Check sheet for the drawn part. Datum: minimum x, y, z corner. Units: mm. Give positions to 0.01 mm unless a question says otherwise; leave off trailing zeros. Loops run counter-clockwise (first coordinate to the right, second up) from the corner with the lowest first, then second, coordinate; pieces in that order, holes last. Notation, with made-up numbers: (19.5, 26) - (48.5, 26) arc R28 cw to (48.5, 54) - close; hole circle Ø3 at (43.5, -0.5). An arc over 180 degrees is marked (long way). Use one line per item in the form item = value.
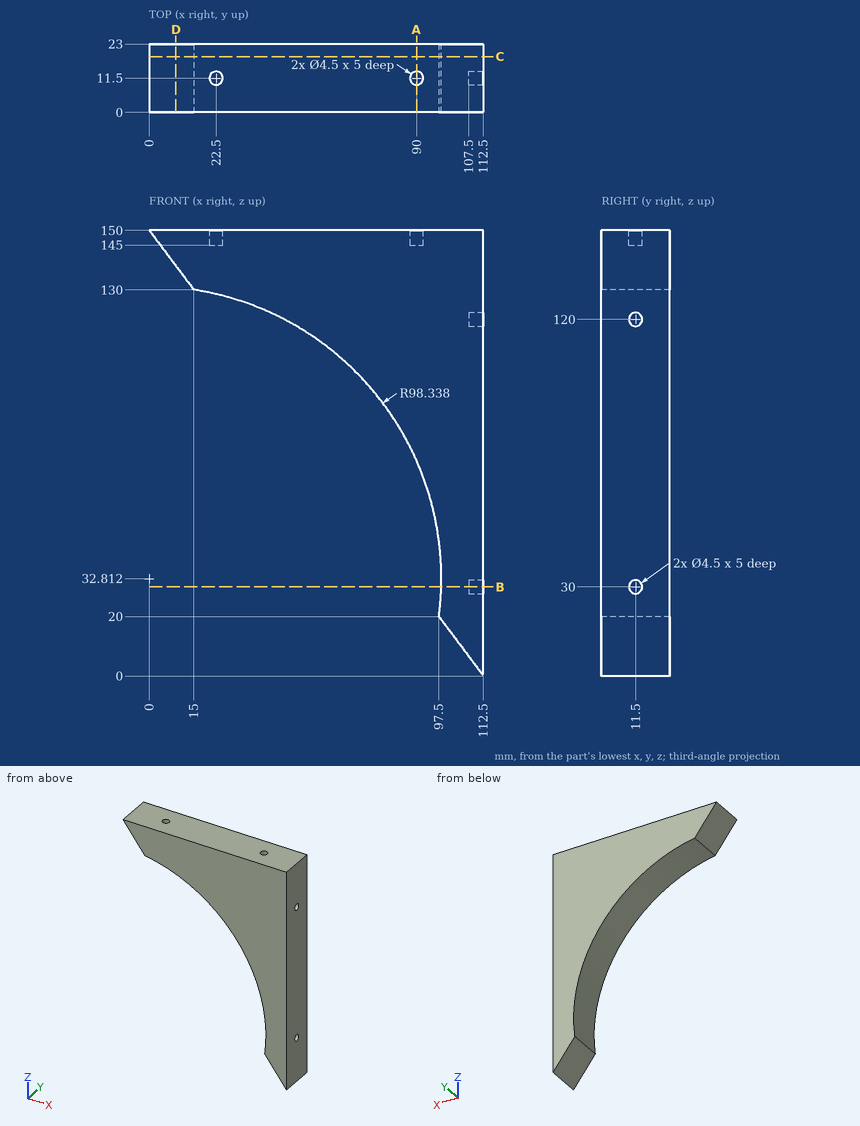
Item 1: Section check B-B on z = 30. Record the boundary of the cut face in (x, y), then the cut area to 3 significant figures.
Answer block:
outline = (98.3, 0) - (112.5, 0) - (112.5, 9.25) - (107.5, 9.25) - (107.5, 13.75) - (112.5, 13.75) - (112.5, 23) - (98.3, 23) - close
area = 304 mm2
Item 2: Gauge pin test, flat ends, axial feed: P1, Ø1, axis at x = 24, y = 13.5, coming from the -Z side; P2, Ø2.5, axis at y = 11.5, z = 120, coming from the +X side; P3, Ø4, axis at x = 90, y = 11.5, coming from the +Z side. Record the tip position at first contact, or that the pin passes through.
Answer block:
P1 = 128.05
P2 = 107.5
P3 = 145
Item 3: Section check A-A on x = 90. Record the boundary of the cut face in (y, z), then the cut area to 3 significant figures.
Answer block:
outline = (0, 72.44) - (23, 72.44) - (23, 150) - (13.75, 150) - (13.75, 145) - (9.25, 145) - (9.25, 150) - (0, 150) - close
area = 1,760 mm2
Item 4: Section check C-C on y = 18.75. Record the boundary of the cut face in (x, z).
Answer block:
outline = (0, 150) - (15, 130) arc R98.34 cw to (97.5, 20) - (112.5, 0) - (112.5, 150) - close
Item 5: Section check D-D on x = 9. Record the boundary of the cut face in (y, z).
Answer block:
outline = (0, 138) - (23, 138) - (23, 150) - (0, 150) - close
Item 6: Thickness scan on L1, parallel to X at y = 11.5, z = 147; L2, parallel to X at y = 11.5, z = 149; L3, parallel to Z at x = 54, y = 11.75. Record the ranges inside material, lowest first.
Answer block:
L1 = 2.25 to 20.25, 24.75 to 87.75, 92.25 to 112.5
L2 = 0.75 to 20.25, 24.75 to 87.75, 92.25 to 112.5
L3 = 115 to 150
